Study the drawing (mm; zero at the part's minimum x, y, z) and answer. A direction names the side the tool comes from. Coordinates: 2 decimals unless noted, no trailing zeros. Loops run counter-clockwise (first coordinate to the right, second up) from the corner with the lowest first, then second, coordinate; pieces in that order, holes last. Notation, with made-up numbers: (69, 25.5) - (96, 25.5) arc R21 cw to (96, 45.5) - close; hole circle Ø5 at (62.5, 30). An arc over 180 degrees is marked (long way). Put each result on its own line as item: value.
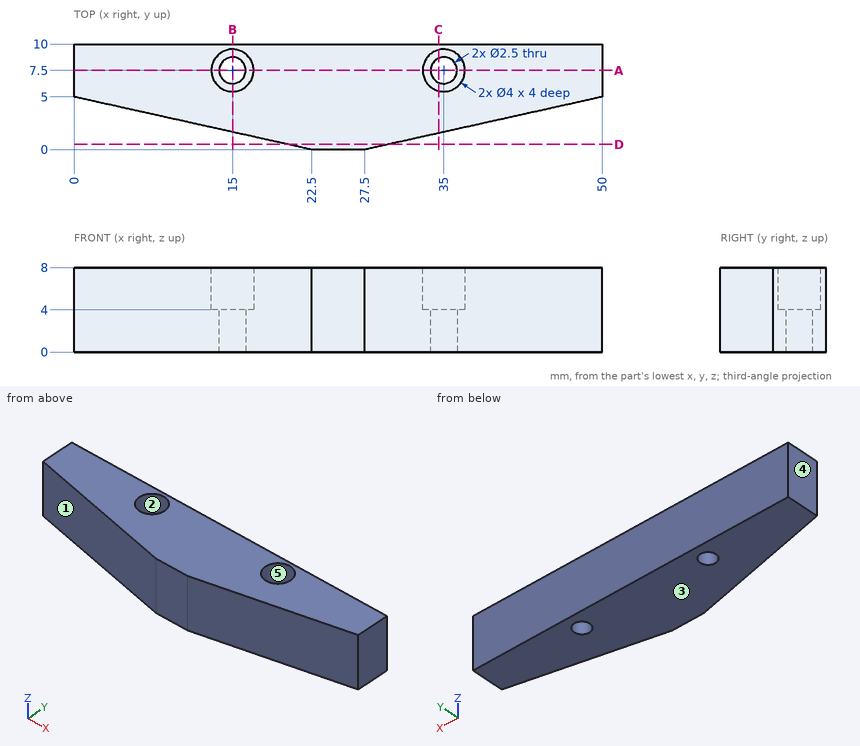
1) For a pull along X with two mould halves and no side action, classify the marked faces 1, 2 and 3 as pulls with the +X half, pulls with the -X half, needs draft (parallel to the pull), parting line crosses it, or undercut.
Found:
face 1: pulls with the -X half
face 2: undercut
face 3: needs draft
2) The part is cut by section C-C (x = 34.5). Give the vertices of the cut face in (y, z).
Found:
outline: (1.56, 0) - (6.35, 0) - (6.35, 4) - (5.56, 4) - (5.56, 8) - (1.56, 8) - close; (8.65, 0) - (10, 0) - (10, 8) - (9.44, 8) - (9.44, 4) - (8.65, 4) - close
3) Each of these flat-tipped pins is pushed along its axis until it touches: pin 1 (1.5 mm diameter, centred on x = 11, z = 6.5, fed in from -Y); pin 2 (2 mm diameter, centred on x = 35, y = 7, fed in from +Z); pin 3 (2 mm diameter, centred on x = 19, z = 1, fed in from -Y). Where does it stop, or does it pass through?
Found:
pin 1: stops at y = 2.39
pin 2: stops at z = 4
pin 3: stops at y = 0.56
4) Straight lines are drawn through the part: L1, parallel to X at y = 7, z = 3.5; L2, parallel to Y at x = 4.5, z = 6.25; L3, parallel to Y at x = 15, z = 1.75. For each, find the intervals that lie inside material, in ascending order. Write a range as [from, to].
Found:
L1: x = [0, 13.85], [16.15, 33.85], [36.15, 50]
L2: y = [4, 10]
L3: y = [1.67, 6.25], [8.75, 10]
5) The part is cut by section B-B (x = 15). Give the vertices of the cut face in (y, z).
Found:
outline: (1.67, 0) - (6.25, 0) - (6.25, 4) - (5.5, 4) - (5.5, 8) - (1.67, 8) - close; (8.75, 0) - (10, 0) - (10, 8) - (9.5, 8) - (9.5, 4) - (8.75, 4) - close
6) The part is cut by section A-A (y = 7.5). Give the vertices of the cut face in (x, z), and give its area (3 significant figures).
Found:
outline: (0, 0) - (13.75, 0) - (13.75, 4) - (13, 4) - (13, 8) - (0, 8) - close; (16.25, 0) - (33.75, 0) - (33.75, 4) - (33, 4) - (33, 8) - (17, 8) - (17, 4) - (16.25, 4) - close; (36.25, 0) - (50, 0) - (50, 8) - (37, 8) - (37, 4) - (36.25, 4) - close
area: 348 mm^2
7) For the marked faces 4 and 5, determine the directions among +Z, -Z, +X, -X, +Y, -Y from which every point of the face is accessible in a straight line to the end or side of a thin tool.
Found:
face 4: +Z, -Z, -X, +Y, -Y
face 5: +Z
8) The part is cut by section D-D (y = 0.5). Give the vertices of the cut face in (x, z).
Found:
outline: (20.25, 0) - (29.75, 0) - (29.75, 8) - (20.25, 8) - close
